Part model, mm, in its own coordinate system. A direction names the side the tool comes from. Coordinates: 2 decimals unless noted, no trailing zeros. Write each loop counter-clockwise with the first axis right and the second up, starting at its lowest first coordinate (ties: lowest second). Pieces come first, ordered by that corner, then holes. Notation, with made-up numbers: (41, 34) -> (92, 34) arc R18 cw to (92, 44) -> close; hole circle Ø5 at (21, -1). An arc over 180 degrees is marked (long way). Write item = value, one per line.
Autodesk Inventor part; units mm, degrees
ref_plane "YZ Plane" through (0, 0, 0) normal (1, 0, 0) x (0, 1, 0)
ref_plane "XZ Plane" through (0, 0, 0) normal (0, 1, 0) x (-1, 0, 0)
ref_plane "XY Plane" through (0, 0, 0) normal (0, 0, 1) x (1, 0, 0)
sketch "Sketch1" plane through (0, 0, 0) normal (0, 0, 1) x (1, 0, 0)
  circle A0 centre (0, 0) radius 35
  dimension "d0" = 70
extrude "Extrusion1" add sketch "Sketch1" along normal mid plane 3
sketch "Sketch2" plane through (0, 0, 1.5) normal (0, 0, 1) x (1, 0, 0)
  circle A0 centre (0, 0) radius 26
  circle A1 centre (0, 0) radius 24.5
  dimension "d3" = 52
  dimension "d4" = 49
extrude "Extrusion2" add sketch "Sketch2" along normal blind 2
sketch "Sketch3" plane through (0, 0, -1.5) normal (0, 0, -1) x (-1, 0, 0)
  circle A0 centre (0, 0) radius 24.5
  dimension "d7" = 49
extrude "Extrusion3" cut sketch "Sketch3" against normal through all
sketch "Sketch5" plane through (0, 0, -1.5) normal (0, 0, -1) x (-1, 0, 0)
  circle A0 centre (0, 30) radius 2
  point P0 (0, 0)
  dimension "d17" = 4
  dimension "d18" = 30
extrude "Extrusion5" cut sketch "Sketch5" against normal through all
pattern_circular "Circular Pattern2" count 4 over 360 about axis through (0, 0, -10) along (0, 0, 1) of "Extrusion5"
thread "Thread1"
thread "Thread2"
thread "Thread3"
thread "Thread4"
properties part number "Flantza_Forea1"
Q1. Probe line 1 (Y direction, x = 0, z = -0.7); line 2 (Z direction, x = -1, y = 27.5); line 3 (Y direction, x = -7, z = 0). List the from-to ranges inside material, lowest first. Write a range as from..to.
Model answer:
line_1 = -35..-32, -28..-24.5, 24.5..28, 32..35
line_2 = -1.5..1.5
line_3 = -34.29..-23.48, 23.48..34.29
Q2. Saw through at C-C on y = 30. Give the cut face in (x, z).
Model answer:
outline = (-18.03, -1.5) -> (-2, -1.5) -> (-2, 1.5) -> (-18.03, 1.5) -> close; (2, -1.5) -> (18.03, -1.5) -> (18.03, 1.5) -> (2, 1.5) -> close
Q3. Mould opens along X. For faces 3 (the face through (-17.5, 17.5, 3.5)), 4 (the face through (0, -28, 0)), 5 (the face through (-28, 21, 0)) say: released by +X, released by -X, zero draft, split by the parting line, or undercut.
Model answer:
face_3 = zero draft
face_4 = undercut
face_5 = split by the parting line
Q4. Which spindle directions (+Z, -Z, +X, -X, +Y, -Y) get a long thin tool onto all of the face, cutting with end or side? Do faces 1 (the face through (-13, 21, -1.5)), 2 (the face through (-20.633, 15.821, 2.486)). Say none if no direction does.
Model answer:
face_1 = -Z, +X, -X, +Y, -Y
face_2 = +Z
Q5. Pin check, flat tips, straight feed: pin 1 (5 mm diameter, centred on x = 14.5, y = -18, fed in from -Z); pin 2 (4.5 mm diameter, centred on x = 0, y = -30, fed in from +Z). Stop position of each tip, or through.
Model answer:
pin_1 = -1.5
pin_2 = 1.5
Q6. Saw through at A-A on x = 0. Give the cut face in (y, z), and give its area (3 significant figures).
Model answer:
outline = (-35, -1.5) -> (-32, -1.5) -> (-32, 1.5) -> (-35, 1.5) -> close; (-28, -1.5) -> (-24.5, -1.5) -> (-24.5, 3.5) -> (-26, 3.5) -> (-26, 1.5) -> (-28, 1.5) -> close; (24.5, -1.5) -> (28, -1.5) -> (28, 1.5) -> (26, 1.5) -> (26, 3.5) -> (24.5, 3.5) -> close; (32, -1.5) -> (35, -1.5) -> (35, 1.5) -> (32, 1.5) -> close
area = 45.0 mm²
